Work out the finished part from the listing and answer in its coordinate system (mm). Face numbers are marked on the shaded views. A direction names the side the tool comes from. Coordinates: 2 decimals unless noted, no trailing zeros. Order: outer loops, then holes, each group sorted by start corner. A loop starts at its lowest first (then second) coordinate and runs counter-clockwise, first axis right, second up. Notation, with made-up numbers: (13.25, -6) -> (24.25, -6) arc R9 cw to (24.25, 2) -> close; hole circle Ø9 at (43, 67). An arc over 180 degrees is marked (long way). Use one line per item in the form item = value.
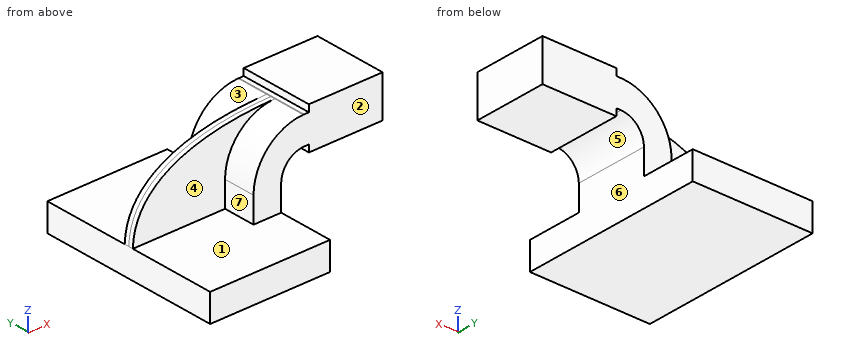
from build123d import *

# Parameters (mm, degrees)
F1_DEPTH = 63.5
F0_W     = 25.4
F0_H     = 19.05
F0_H_2   = 4.7498
F0_H_3   = 4.7752
F2_DEPTH = 25.4
F3_DEPTH = 3.175


with BuildPart() as f1:
    # F0 (on Front) → F1 (new body, symmetric)
    with BuildSketch(Plane.XZ):
        Polygon((41.275, -9.525), (41.275, 9.525), (22.225, 9.525), (-41.275, 9.525), (-41.275, -9.525), align=None)
    extrude(amount=F1_DEPTH, both=True)

    # F0 (on Front) → F2 (join, symmetric)
    with BuildSketch(Plane.XZ):
        with BuildLine():
            Line((22.225, 9.525), (41.275, 9.525))
            Line((41.275, 9.525), (41.275, 27.0002))
            ThreePointArc((41.275, 27.0002), (45.9246798487, 38.2255201513), (57.15, 42.8752))
            Line((57.15, 42.8752), (60.325, 42.8752))
            Line((60.325, 42.8752), (60.325, 61.9252))
            Line((60.325, 61.9252), (57.15, 61.9252))
            add(Edge.make_bspline(
                [(56.4749540352, 61.918675596), (56.6996080487, 61.9210846783), (56.9246234605, 61.9232595365), (57.15, 61.9252)],
                knots=[111.1038560416, 111.1038560416, 111.1038560416, 111.1038560416, 111.5045361635, 111.5045361635, 111.5045361635, 111.5045361635], degree=3))
            ThreePointArc((56.4749540352, 61.918675596), (32.2167731198, 51.4560750066), (22.225, 27.0002))
            Line((22.225, 27.0002), (22.225, 9.525))
        make_face()
        with Locations((73.025, 52.4002)):
            Rectangle(F0_W, F0_H)
        Polygon((85.725, 61.9252), (85.725, 42.8752), (85.725, 38.1), (111.125, 38.1), (111.125, 66.675), (85.725, 66.675), align=None)
        with Locations((73.025, 64.3001)):
            Rectangle(F0_W, F0_H_2)
        with Locations((73.025, 40.4876)):
            Rectangle(F0_W, F0_H_3)
    extrude(amount=F2_DEPTH, both=True)

    # F0 (on Front) → F3 (join, symmetric)
    with BuildSketch(Plane.XZ):
        with BuildLine():
            Line((-41.275, 9.525), (22.225, 9.525))
            Line((22.225, 9.525), (22.225, 27.0002))
            ThreePointArc((22.225, 27.0002), (32.2167731198, 51.4560750066), (56.4749540352, 61.918675596))
            add(Edge.make_bspline(
                [(-41.275, 9.525), (-40.3253856931, 42.5734618465), (-5.8189452735, 61.2506655739), (56.4749540352, 61.918675596)],
                knots=[0, 0, 0, 0, 111.1038560416, 111.1038560416, 111.1038560416, 111.1038560416], degree=3))
        make_face()
    extrude(amount=F3_DEPTH, both=True)


solid = f1.part
(1) Which of the six approach directions +Z, -Z, +X, -X, +Y, -Y give full straight-line access (tool end or side, diameter ignored) to the marked faces 1, 2 and 3?
Data:
face_1 = +Z, -X, -Y
face_2 = +Z, +X, -X, -Y
face_3 = +Z, -X, +Y
(2) Section B-B on z = 6 is taken. Write down the section's boundary in (x, y) (3 decimals).
Data:
outline = (-41.275, -63.5) -> (41.275, -63.5) -> (41.275, 63.5) -> (-41.275, 63.5) -> close
(3) Section A-A on x = 64 is taken. Write down the section's boundary in (y, z) (3 decimals), plus the area to 3 significant figures.
Data:
outline = (-25.4, 38.1) -> (25.4, 38.1) -> (25.4, 66.675) -> (-25.4, 66.675) -> close
area = 1,450 mm²
(4) The mould has two halves that part along X. Classify the marked faces 4, 5, 6 and 7: released by +X, released by -X, zero draft, split by the parting line, or undercut.
Data:
face_4 = zero draft
face_5 = undercut
face_6 = released by +X
face_7 = released by -X
(5) Straight lines are drawn through the part: line 1 along Z through (x, y) = (-4.5, 5.5) (3 decimals); line 2 along X through (y, z) = (-17.5, -4) (3 decimals); line 3 along Y through (x, z) = (15, 13) (3 decimals). For each, find the intervals that lie inside material, in ascending order.
Data:
line_1 = -9.525 to 9.525
line_2 = -41.275 to 41.275
line_3 = -3.175 to 3.175
(6) Each of these flat-tipped pins is pushed along its axis until it touches: P1, Ø2.5, axis at y = -0.5, z = 65, coming from the -X side (3 decimals); P2, Ø10, axis at x = 21, z = 54.5, coming from the +Y side (3 decimals); P3, Ø1, axis at x = 59, y = 11, coming from the +Z side. Where does it stop, or does it pass through?
Data:
P1 = 60.325
P2 = 3.175
P3 = 61.93
